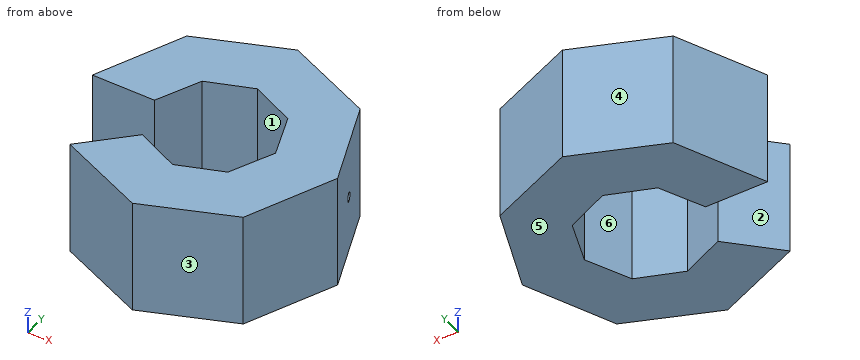
```python
from build123d import *

# Parameters (mm, degrees)
BOSS_EXTRUDE1_DEPTH = 10
SKETCH2_R           = 0.4
CUT_EXTRUDE1_DEPTH  = 602


with BuildPart() as part:
    # Sketch1 → Boss-Extrude1 (new body)
    with BuildSketch(Plane.XY):
        Polygon((-3.979511218, -3.667807567), (-0.220407765, -5.407470971), (3.667807567, -3.979511218), (5.407470971, -0.220407765), (3.979511218, 3.667807567), (0.220407765, 5.407470971), (-3.667807567, 3.979511218), (-5.407470971, 0.220407765), (-10.821084843, 0.247811103), (-7.476433561, 7.826891384), (0.247811103, 10.821084843), (7.826891384, 7.476433561), (10.821084843, -0.247811103), (7.476433561, -7.826891384), (-0.247811103, -10.821084843), (-7.826891384, -7.476433561), align=None)
    extrude(amount=-BOSS_EXTRUDE1_DEPTH)

    # Sketch2 → Cut-Extrude1 (cut)
    with BuildSketch(Plane(origin=(9.323988114, 3.614311229, 0), x_dir=(0, 0, -1), z_dir=(0.9323988113551661, 0.361431122876093, 0))):
        with Locations(Location((5, 0, 0), (0, 0, 90))):
            Circle(SKETCH2_R)
    extrude(amount=-CUT_EXTRUDE1_DEPTH, mode=Mode.SUBTRACT)


solid = part.part
```
Source: CAD feature listing. Evaluate the final solid. Frame: model axes, mm. Face numbers are marked on the shaded views. A direction names the side the tool comes from. Round coordinates to 2 decimals unless told otherwise and drop trailing zeros. Loops run counter-clockwise (first coordinate to the right, second up) from the corner with the lowest first, then second, coordinate; pieces in that order, holes last.
(1) Section query C-C (z = -8.25). Output: boundary loops of the cut face in (x, y), and give its area (3 significant figures).
From the geometry:
outline: (-10.82, 0.25) - (-5.41, 0.22) - (-3.67, 3.98) - (0.22, 5.41) - (3.98, 3.67) - (5.41, -0.22) - (3.67, -3.98) - (-0.22, -5.41) - (-3.98, -3.67) - (-7.83, -7.48) - (-0.25, -10.82) - (7.48, -7.83) - (10.82, -0.25) - (7.83, 7.48) - (0.25, 10.82) - (-7.48, 7.83) - close
area: 217 mm2
(2) Pull-direction query (Y, two-part tool) for the marked faces 4, 5 and 6; classes: +Y half, -Y half, draft (parallel to the pull), parting line (faces both ways), or undercut.
From the geometry:
face 4: +Y half
face 5: draft
face 6: undercut
(3) Section query D-D (x = -8.25). Output: boundary loops of the cut face in (y, z).
From the geometry:
outline: (0.23, -10) - (6.07, -10) - (6.07, 0) - (0.23, 0) - close
(4) Section query B-B (x = 2.75). Output: boundary loops of the cut face in (y, z), and give its area (3 significant figures).
From the geometry:
outline: (-9.66, -10) - (-4.32, -10) - (-4.32, 0) - (-9.66, 0) - close; (4.24, -10) - (9.72, -10) - (9.72, 0) - (4.24, 0) - close
area: 108 mm2
(5) Section query A-A (y = -4.5). Output: boundary loops of the cut face in (x, z), and give its area (3 significant figures).
From the geometry:
outline: (-4.82, -10) - (-2.18, -10) - (-2.18, 0) - (-4.82, 0) - close; (2.25, -10) - (8.94, -10) - (8.94, 0) - (2.25, 0) - close
area: 93.3 mm2
(6) Access query for the marked faces 1, 2 and 3. Directions: +Z, -Z, +X, -X, +Y, -Y. A direction counts if a zero-diameter tool reaches every point of the face in a straight line with its end or side. Return the directions, or none.
From the geometry:
face 1: +Z, -Z
face 2: +Z, -Z, -X
face 3: +Z, -Z, +X, -Y
(7) Material intervals for probe 1 along Y at (x, z) = (-7.5, -3.25); probe 2 along Y at (x, z) = (-6.75, -1.25); probe 3 along X at (y, z) = (-7.5, -8.5), sorted ascending.
From the geometry:
probe 1: y = -7.62 to -7.15, 0.23 to 7.77
probe 2: y = -7.95 to -6.41, 0.23 to 8.11
probe 3: x = -7.77 to 7.62
(8) Contact query for flat-ended pins moving along their axis: pin 1 Ø5 at (y, z) = (3, -2.5) entering from +X; pin 2 Ø2 at (y, z) = (-5, -4) entering from +X; pin 3 Ø5 at (x, z) = (3.5, -1) entering from -Y. Output: stop coordinate, or through.
From the geometry:
pin 1: stops at x = 10.53
pin 2: stops at x = 9.17
pin 3: stops at y = -10.34
